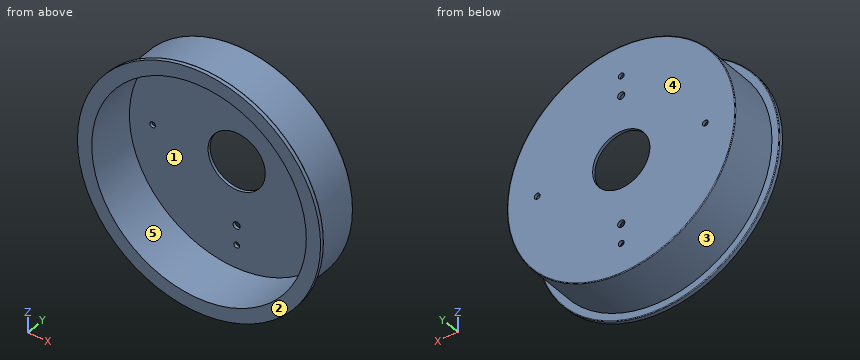
```python
from build123d import *

# Parameters (mm, degrees)
F0_R      = 79.8
F0_R_2    = 20
F1_DEPTH  = 5
F2_R      = 79.8
F2_R_2    = 75
F3_DEPTH  = 30
F4_R      = 85
F4_R_2    = 75
F5_DEPTH  = 3
F7_D      = 5
F7_DEPTH  = 25
F7_TIP    = 1.5021515476
F8_R      = 0.5
F9_DEPTH  = 3
F11_D     = 4
F11_DEPTH = 25
F11_TIP   = 1.2017212381


with BuildPart() as f1:
    # F0 (on Front) → F1 (new body)
    with BuildSketch(Plane.XZ):
        Circle(F0_R)
        Circle(F0_R_2, mode=Mode.SUBTRACT)
    extrude(amount=F1_DEPTH)

    # F2 (on face) → F3 (join)
    with BuildSketch(Plane.XZ.offset(5)):
        Circle(F2_R)
        Circle(F2_R_2, mode=Mode.SUBTRACT)
    extrude(amount=F3_DEPTH)

    # F4 (on face) → F5 (join)
    with BuildSketch(Plane.XZ.offset(35)):
        Circle(F4_R)
        Circle(F4_R_2, mode=Mode.SUBTRACT)
    extrude(amount=F5_DEPTH)

    # F7
    with Locations(Plane(origin=(0, 0, 0), x_dir=(-1, 0, 0), z_dir=(0, 1, 0))):
        with Locations((0, 45), (0, -45)):
            Hole(F7_D / 2, depth=F7_DEPTH)
            with Locations((0, 0, -(F7_DEPTH + F7_TIP / 2))):  # 118° drill point
                Cone(0, F7_D / 2, F7_TIP, mode=Mode.SUBTRACT)

    # F8
    f8_edges = [f1.edges().sort_by_distance(p)[0] for p in [
        (-79.8, 0, 0),
        (-85, -35, 0),
    ]]
    fillet(f8_edges, radius=F8_R)

    # F9 (cut): a face of the model
    f9_faces = [f1.faces().sort_by_distance(p)[0] for p in [
        (-72.8786796564, -5, 0),
    ]]
    extrude(f9_faces, amount=-F9_DEPTH, mode=Mode.SUBTRACT)

    # F11
    with Locations(Plane(origin=(0, 0, 0), x_dir=(-1, 0, 0), z_dir=(0, 1, 0))):
        with Locations((-58.75, 0), (0, 58.75), (58.75, 0), (0, -58.75)):
            Hole(F11_D / 2, depth=F11_DEPTH)
            with Locations((0, 0, -(F11_DEPTH + F11_TIP / 2))):  # 118° drill point
                Cone(0, F11_D / 2, F11_TIP, mode=Mode.SUBTRACT)


solid = f1.part
```
Geometry check sheet. Reference: the model listing, model coordinates, mm. Face numbers are marked on the shaded views. A direction names the side the tool comes from. Give positions to 0.01 mm unless a question says otherwise; leave off trailing zeros. Loops run counter-clockwise (first coordinate to the right, second up) from the corner with the lowest first, then second, coordinate; pieces in that order, holes last. Notation, with made-up numbers: (61, 84.25) - (98, 84.25) arc R22 cw to (98, 101.25) - close; hole circle Ø11 at (-5.75, 31.5). An arc over 180 degrees is marked (long way). Use CSV: the item, a comma, the result in double quotes. Start each with the question number.
Q1. Access from +Z, -Z, +X, -X, +Y, -Y to the whole of each face (thin tool, end or side, straight path). Record for the marked faces 1 and 2.
Q2. Section check A-A, the plane y = -10.5. Record the cut outline in (x, z), and give its area (3 significant figures).
Q3. Release check for a two-part mould opening along X. For the marked faces 3, 4 and 5 record: +X half, -X half, draft (parallel to the pull), parting line (faces both ways), or undercut.
Q4. Scan lines: probe 1 along Z at (x, y) = (0, -0.7); probe 2 along Y at (x, z) = (36.5, -55); probe 3 along Z at (x, y) = (-21, -3). Record each from-to range of solid material in increasing order. Write a range as from..to.
Q5. Go/stop test with flat-tipped pins: pin 1 Ø10 at (x, z) = (13.5, 9) entering from +Y; pin 2 Ø4 at (x, z) = (0, 45) entering from +Y; pin 3 Ø3 at (x, z) = (-25.5, -9.5) entering from -Y; pin 4 Ø3 at (y, z) = (-31, -50) entering from +X. Record where each tip stops, or that it passes through.
Findings below:
1,face 1,"-Y"
1,face 2,"+Z, -Z, +X, -X, -Y"
2,outline,"circle Ø159.6 at (0, 0); hole circle Ø150 at (0, 0)"
2,area,"2,330 mm^2"
3,face 3,"parting line"
3,face 4,"draft"
3,face 5,"undercut"
4,probe 1,"z = -79.8..-60.75, -56.75..-47.5, -42.5..-20, 20..42.5, 47.5..56.75, 60.75..79.8"
4,probe 2,"y = -2..0"
4,probe 3,"z = -76.99..-72, 72..76.99"
5,pin 1,"stops at y = 0"
5,pin 2,"passes through"
5,pin 3,"stops at y = -2"
5,pin 4,"stops at x = 63.37"
